Input: part model. Units: mm. Frame: model coordinates. Round coordinates to 2 decimals unless told otherwise and drop trailing zeros. Order: outer loops, then holes, each group sorted by start corner. A loop starts at its lowest first (then second) coordinate and runs counter-clockwise, first axis right, second up. Notation, with made-up numbers: (35.25, 19) -> (82.25, 19) arc R26 ccw to (82.25, 42) -> close; hole circle Ø3 at (-38.5, 2.25). An arc over 180 degrees is marked (long way). Use a Markdown table: item, result.
Autodesk Fusion 360 part; units mm, degrees
sketch "草图1" plane through (0, 0, 0) normal (0, 0, 1) x (1, 0, 0)
  line L0 (0, 0) -> (60, 0)
  line L1 (60, 0) -> (60, -100)
  line L2 (60, -100) -> (0, -100)
  line L3 (0, -100) -> (0, 0)
  dimension "d1" = 60
  dimension "d2" = 100
extrude "拉伸1" add sketch "草图1" along normal blind 5
sketch "草图2" plane through (0, 0, 5) normal (0, 0, 1) x (-1, 0, 0)
  line L0 (0, 100) -> (-60, 100)
  line L1 (-60, 100) -> (-60, 0)
  line L2 (-60, 0) -> (0, 0)
  line L3 (0, 0) -> (0, 100)
  circle A0 centre (-8, 8) radius 1.6
  circle A1 centre (-52, 8) radius 1.6
  circle A2 centre (-8, 92) radius 1.6
  circle A3 centre (-52, 92) radius 1.6
  dimension "d5" = 3.2
  dimension "d6" = 8
  dimension "d7" = 8
  dimension "d14" = -44
  dimension "d15" = 84
extrude "拉伸2" cut sketch "草图2" against normal blind 5 contours A0 | A1 | A2 | A3
1) Ray query, probe 1 along Y at (x, z) = (52, 2.35); probe 2 along X at (y, z) = (-8, 1.45). Return the intervals inside material, ascending.
Answer key:
| item | result |
|---|---|
| probe 1 | y = -100 to -93.6, -90.4 to -9.6, -6.4 to 0 |
| probe 2 | x = 0 to 6.4, 9.6 to 50.4, 53.6 to 60 |
2) Draft query along X for faces 1 (the face through (9.27, -7.03, 2.54)), 2 (the face through (60, -49, 2)), 3 (the face through (30, -49, 5)). Return one class per face: released by +X, released by -X, zero draft, split by the parting line, or undercut.
Answer key:
| item | result |
|---|---|
| face 1 | undercut |
| face 2 | released by +X |
| face 3 | zero draft |
3) Cut plane A-A on x = 52. Return loops of the section in (y, z).
Answer key:
| item | result |
|---|---|
| outline | (-100, 0) -> (-93.6, 0) -> (-93.6, 5) -> (-100, 5) -> close; (-90.4, 0) -> (-9.6, 0) -> (-9.6, 5) -> (-90.4, 5) -> close; (-6.4, 0) -> (0, 0) -> (0, 5) -> (-6.4, 5) -> close |
4) Cut plane B-B on y = -92. Return loops of the section in (x, z).
Answer key:
| item | result |
|---|---|
| outline | (0, 0) -> (6.4, 0) -> (6.4, 5) -> (0, 5) -> close; (9.6, 0) -> (50.4, 0) -> (50.4, 5) -> (9.6, 5) -> close; (53.6, 0) -> (60, 0) -> (60, 5) -> (53.6, 5) -> close |
